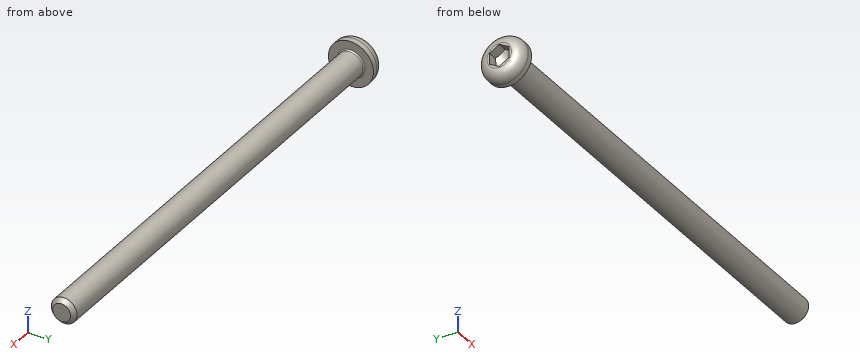
Autodesk Inventor part; units mm, degrees
ref_plane "Work Plane1" through (29, 0, 0) normal (0, -1, 0) x (1, 0, 0)
ref_plane "YZ Plane" through (0, 0, 0) normal (1, 0, 0) x (0, 1, 0)
ref_plane "XZ Plane" through (0, 0, 0) normal (0, 1, 0) x (-1, 0, 0)
sketch "Sketch1" plane through (0, 0, 0) normal (0, 0, 1) x (1, 0, 0)
  line L0 (0, 0) -> (35, 0)
  line L1 (35, 0) -> (35, 1)
  line L2 (35, 1) -> (30.5, 1)
  line L3 (30.5, 1) -> (30.1932, 1)
  line L4 (30.1932, 1) -> (0, 1)
  line L5 (0, 1) -> (0, 1.75)
  line L6 (0, 1.75) -> (-1.2, 1.75)
  line L7 (-1.2, 1.75) -> (-1.2, 0.866)
  line L8 (-1.2, 0.866) -> (-0.5, 0.866)
  line L9 (-0.5, 0.866) -> (0, 0)
  line L10 (-8.44, 0) -> (42.24, 0)
  line L11 (0, -0.35) -> (0, 2.1)
  line L12 (30.5, 1) -> (0, 1) construction
  dimension "d1" = 4.5
  dimension "d2" = 0.3068
  dimension "d3" = 1.2
  dimension "d4" = 0.7
  dimension "d5" = 60
  dimension "d6" = 2
  dimension "d7" = 2
  dimension "d8" = 1.7321
  dimension "d9" = 3.5
  dimension "d26" = 35
revolve "Body" add sketch "Sketch1" angle 360 about axis through (0, 0, 0) along (1, 0, 0)
sketch "Sketch2" plane through (-1.2, 0, 0) normal (-1, 0, 0) x (0, 0, 1)
  circle A0 centre (0, 0) radius 0.866
  line L0 (0, -2.45) -> (0, 2.45)
  line L1 (-2.45, 0) -> (2.45, 0)
  line L2 (0.866, 0) -> (0.433, -0.75)
  line L3 (0.433, -0.75) -> (-0.433, -0.75)
  line L4 (-0.433, -0.75) -> (-0.866, 0)
  line L5 (-0.866, 0) -> (-0.433, 0.75)
  line L6 (-0.433, 0.75) -> (0.433, 0.75)
  line L7 (0.433, 0.75) -> (0.866, 0)
extrude "Slot" add sketch "Sketch2" against normal up to next contours L7 A0 | A0 L2 | L6 L0 A0 | A0 L0 L3 | L0 L6 A0 | A0 L3 L0 | L4 A0 | A0 L5
fillet "Fillet1" radius 0.8 1 edges at (-1.2, -1.75, 0)
chamfer "Chamfer1" distance 0.3067 distance2 0.3067 1 edges at (35, -1, 0) measured on face at (35, 0.3333, 0.4421)
ref_plane "Work Plane1" through (29, 0, 0) normal (0, -1, 0) x (1, 0, 0)
fillet "Fillet2" radius 0.1 1 edges at (0, -1, 0)
thread "Thread2"
equation "\"d15\" = -0.5 * SPD + 0.5 * GD"
equation "\"d16\" = GUL"
equation "\"d1\" = GEL"
equation "\"GD\" = NND"
equation "\"NLG\" = 6"
equation "\"GEL\" = 4.5"
equation "\"KOD\" = 5.7"
equation "\"KOH\" = 1.65"
equation "\"INTI\" = 1.04"
equation "\"GAL\" = 0.61345 * PTC"
equation "\"GUL\" = 0.61345 * PTC"
equation "\"BDM\" = NND"
equation "\"SW\" = 2"
equation "\"RR\" = 1.45"
equation "\"SPD\" = NND - 1.2269 * PTC"
equation "\"R\" = 0.3"
equation "\"TOA\" = 30deg"
equation "\"GD1\" = THREADDIA - 1.2269 * PTC"
equation "\"THREADDIA\" = 3"
equation "\"PTC\" = 0.5"
equation "\"NND\" = 3"
equation "\"KOH1\" = 0.2"
equation "\"E0\" = 2.303"
properties part number "ISO 7380-1 - M3 x 6" material "Stainless Steel"
Can you work these out from the model? Positions are in its coordinate system, mm. Give positions to 0.01 mm unless a question says otherwise; leave off trailing zeros. Write each loop counter-clockwise with the first axis right and the second up, starting at its lowest first coordinate (ties: lowest second). Pieces come first, ordered by that corner, then holes. Notation, with made-up numbers: (30, 65) -> (65, 65) arc R32 ccw to (65, 100) -> close; hole circle Ø4 at (87, -17.5). An arc over 180 degrees is marked (long way). Write item = value, one per line.
(1) Suppose I cut it at A-A on x = 31. Write out the boundary of the cut face in (y, z).
Worked out:
outline = circle Ø2 at (0, 0)
(2) I'm going to push flat-ended pins straight in: P1, Ø0.6, axis at x = -1, z = 0, coming from the +Y side; P2, Ø0.8, axis at x = -1, z = 0, coming from the -Y side. Where does each tip first touch, or does it pass through?
Worked out:
P1 = 1.69
P2 = -1.72
(3) I need wall thicknesses on probe 1 along Y at (x, z) = (12, 0.5); probe 2 along Z at (x, y) = (1.5, 0.05); probe 3 along X at (y, z) = (0.25, 1.65). Which ranges of each line are inside material? Lowest first, please. Write a range as from..to.
Worked out:
probe_1 = -0.87..0.87
probe_2 = -1..1
probe_3 = -0.75..0
